from build123d import *

# Parameters (mm, degrees)
SKETCH_1_R          = 14.5
EXTRUDE_1_DEPTH     = 2
SKETCH_2_R          = 7.5
CUT_EXTRUDE_2_DEPTH = 2.5
SKETCH_1_4_R        = 1.75
CUT_EXTRUDE_1_DEPTH = 2.8


with BuildPart() as part:
    # Эскиз1 → Бобышка-Вытянуть1 (new body)
    with BuildSketch(Plane.XY):
        Circle(SKETCH_1_R)
    extrude(amount=EXTRUDE_1_DEPTH)

    # Эскиз2 → section 1 of loft_1
    with BuildSketch(Plane.XY.offset(4.5), mode=Mode.PRIVATE) as loft_1_s1:
        Circle(SKETCH_2_R)
    # loft from a face of the part (loft_1)
    loft([part.faces().sort_by_distance((0, 0, 2))[0], loft_1_s1.sketch])

    # Эскиз2<4> → Вырез-Вытянуть2 (cut)
    with BuildSketch(Plane.XY.offset(4.5)):
        Polygon((0, 3.233161507), (-2.8, 1.616580754), (-2.8, -1.616580754), (0, -3.233161507), (2.8, -1.616580754), (2.8, 1.616580754), align=None)
    extrude(amount=-CUT_EXTRUDE_2_DEPTH, mode=Mode.SUBTRACT)

    # Эскиз1<4> → Вырез-Вытянуть1 (cut)
    with BuildSketch(Plane.XY):
        Circle(SKETCH_1_4_R)
    extrude(amount=CUT_EXTRUDE_1_DEPTH, mode=Mode.SUBTRACT)


solid = part.part
Verification items for the finished model (mm, model axes). A direction names the side the tool comes from. Coordinates: 2 decimals unless noted, no trailing zeros. Write each loop counter-clockwise with the first axis right and the second up, starting at its lowest first coordinate (ties: lowest second). Pieces come first, ordered by that corner, then holes. Notation, with made-up numbers: (-21.5, 78.5) -> (-5.5, 78.5) arc R16 cw to (-5.5, 90.5) -> close; hole circle Ø8 at (70, 77). An arc over 180 degrees is marked (long way). One line per item, written item: value. Start each with the question number.
Q1. Access from +Z, -Z, +X, -X, +Y, -Y to the whole of each face (thin tool, end or side, straight path). Record for faces 4 (the flat face through (-1.3, -1.4, 2)), 5 (the cylindrical face through (1.617, -0.67, 0.986)).
Q2. Cross-section at A-A on z = 3.35. Enter the section's corners in (x, y).
Q3. Go/stop test with a flat-tipped pin: P1, Ø2, axis at y = -7, z = 0.5, coming from the +X side. Record where the tip stops, or that it passes through.
Q4. Thickness scan on L1, parallel to Y at x = 0, z = 1.4; L2, parallel to X at y = -1.5, z = 0.3; L3, parallel to Z at x = 11.25, y = -5.25. Record the ranges inside material, lowest first. Write a range as from..to.
Q5. Mould release check, pull along X, two halves, no side actions. Record for faces 1 (the conical face through (-1.7, -7.65, 4.38)), 2 (the flat face through (2.8, 0, 3)), 3 (the flat face through (3, 0, 4.5)): pulls with the +X half, pulls with the -X half, needs draft (parallel to the pull), parting line crosses it, or undercut.
Checked values:
1. face 4: +Z
1. face 5: +Z, -Z
2. outline: circle Ø21.44 at (0, 0); hole (-2.8, -1.62) -> (0, -3.23) -> (2.8, -1.62) -> (2.8, 1.62) -> (0, 3.23) -> (-2.8, 1.62) -> close
3. P1: stops at x = 13.2
4. L1: y = -14.5..-1.75, 1.75..14.5
4. L2: x = -14.42..-0.9, 0.9..14.42
4. L3: z = 0..2.74
5. face 1: parting line crosses it
5. face 2: undercut
5. face 3: needs draft
